Could you check a few things on this drawing? It's one solid part, dimensions in mm from its lowest x, y, z. Coordinates: 2 decimals unless noted, no trailing zeros. Write each loop counter-clockwise with the first axis right and the second up, starting at its lowest first coordinate (ties: lowest second). Pieces come first, ordered by that corner, then holes. Notation, with made-up numbers: (-26, -29.75) - (2, -29.75) arc R13 cw to (2, -14.75) - close; hole circle Ø4 at (87, 88). An arc over 180 degrees is marked (long way). Answer as a JSON object with one key per item and string values. Group by question number.
1) If we section it at C-C (z = 88): Write out the boundary of the cut face in (x, y), plus the area to 3 significant figures.
2) If we section it at A-A (y = 12.7): Write out the boundary of the cut face in (x, z).
3) Please list where these lines run through material, in increasing order: line 1 along X through (y, z) = (12.7, 43.5); line 2 along Y through (x, z) = (13, 35); line 3 along Y through (x, z) = (12.7, 91).
4) We'd pull the mould along X, two halves only. Please class the marked faces 1, 2 and 3: released by +X, released by -X, zero draft, split by the parting line, or undercut.
5) If we section it at D-D (z = 62): Write out the boundary of the cut face in (x, y).
6) Will these pins go through, and if not, where does the flat tip stop? pin 1 Ø10 at (x, y) = (13, 14) entering from +Z; pin 2 Ø12 at (x, z) = (3, 46) entering from +Y; pin 3 Ø1 at (y, z) = (19.5, 47) entering from -X.
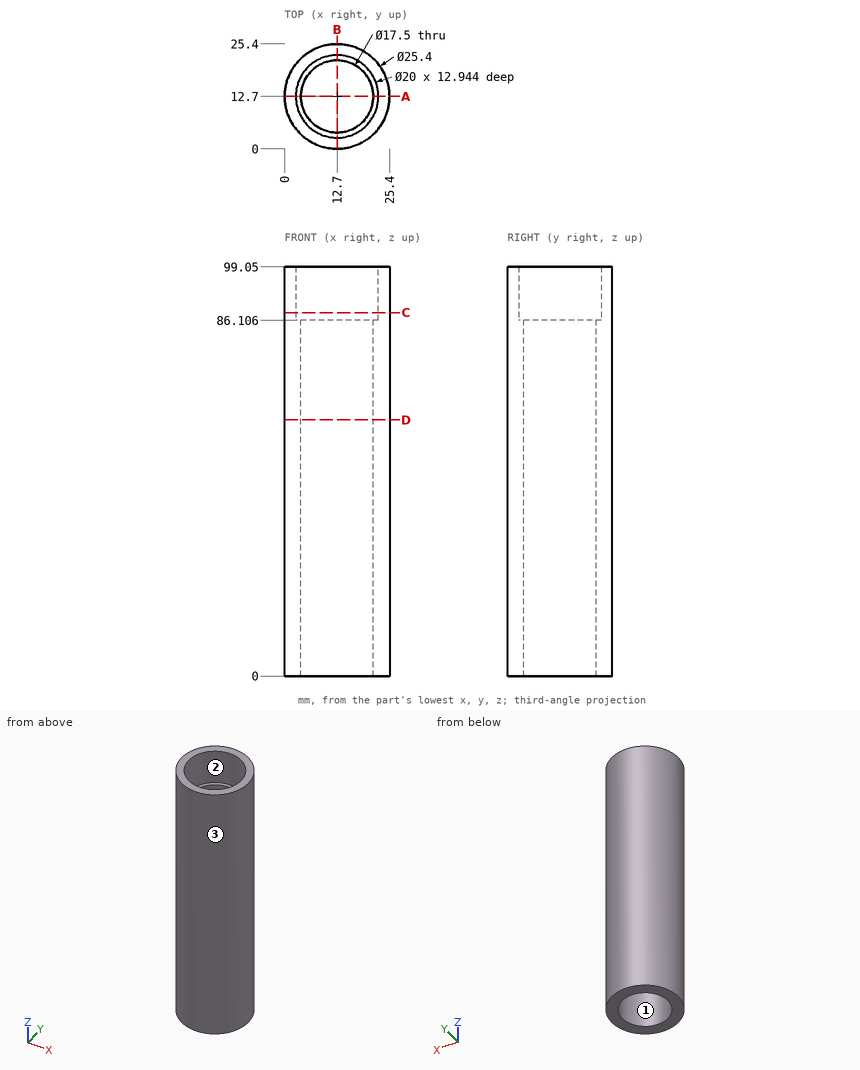
Here are the results:
{
 "1": {"outline": "circle Ø25.4 at (12.7, 12.7); hole circle Ø20 at (12.7, 12.7)", "area": "193 mm²"},
 "2": {"outline": "(0, 0) - (3.95, 0) - (3.95, 86.11) - (2.7, 86.11) - (2.7, 99.05) - (0, 99.05) - close; (21.45, 0) - (25.4, 0) - (25.4, 99.05) - (22.7, 99.05) - (22.7, 86.11) - (21.45, 86.11) - close"},
 "3": {"line 1": "x = 0 to 3.95, 21.45 to 25.4", "line 2": "y = 0 to 3.96, 21.44 to 25.4", "line 3": "y = 0 to 2.7, 22.7 to 25.4"},
 "4": {"face 1": "undercut", "face 2": "undercut", "face 3": "split by the parting line"},
 "5": {"outline": "circle Ø25.4 at (12.7, 12.7); hole circle Ø17.5 at (12.7, 12.7)"},
 "6": {"pin 1": "passes through", "pin 2": "stops at y = 24.85", "pin 3": "stops at x = 1.67"}
}
